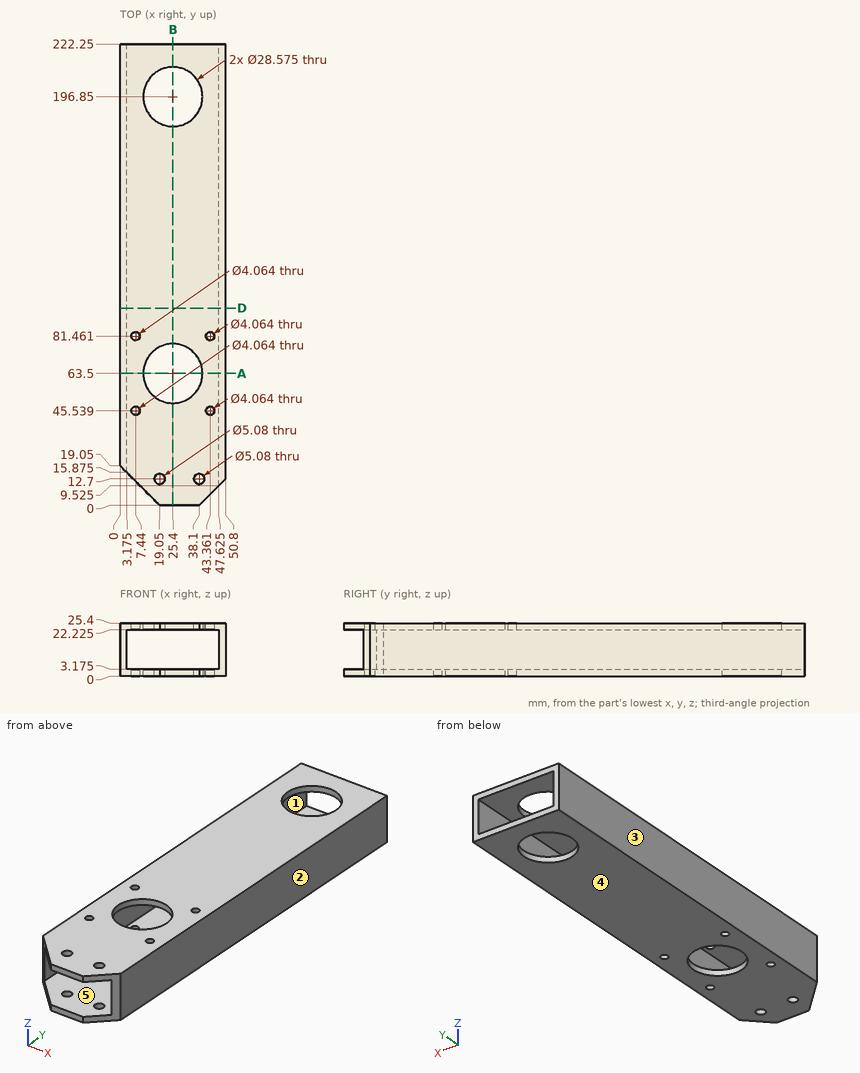
Geometry: see drawing. Coordinates: mm, zero at the bounding-box minimum. A direction names the side the tool comes from. Round coordinates to 2 decimals unless told otherwise and drop trailing zeros. Loops run counter-clockwise (first coordinate to the right, second up) from the corner with the lowest first, then second, coordinate; pieces in that order, holes last. Notation, with made-up numbers: M -22,8.25 L -2,8.25 A21 cw -2,23.25 Z; hole C -10.75,4.25 d1. An arc over 180 degrees is marked long. Use a Markdown table: item, result. Add a question column.
1. Cut plane D-D, the plane y = 95. Output: boundary loops of the cut face in (x, z) (1 decimal).
2. Set-up query: the marked faces 1 and 2. Return all of +Z, -Z, +X, -X, +Y, -Y with unobstructed straight access to the full face (end or side cutting, diameter ignored); none if empty.
3. Contact query for a flat-ended pin moving along its axis: pin 1 (3 mm diameter, centred on x = 44, z = 6.5, fed in from +Y). Output: stop coordinate, or through.
4. Cut plane A-A, the plane y = 63.5. Output: boundary loops of the cut face in (x, z) (1 decimal), and give its area (3 significant figures).
5. Pull-direction query (X, two-part tool) for the marked faces 3, 4 and 5; classes: +X half, -X half, draft (parallel to the pull), parting line (faces both ways), or undercut.
6. Cut plane B-B, the plane x = 25.4. State how many separate pieces and enclosed holes the cut face has, and give its area (3 significant figures).
7. Ray query, line 1 along Z through (x, y) = (6, 137.5) (1 decimal); line 2 along Y through (x, z) = (25.4, 22.9); line 3 along X through (y, z) = (158, 12.5) (1 decimal). Return the intervals inside material, ascending. Write a range as [from, to].
Solution:
| question | item | result |
|---|---|---|
| 1 | outline | M 0,0 L 50.8,0 L 50.8,25.4 L 0,25.4 Z; hole M 3.2,3.2 L 47.6,3.2 L 47.6,22.2 L 3.2,22.2 Z |
| 2 | face 1 | +Y, -Y |
| 2 | face 2 | +Z, -Z, +X, +Y, -Y |
| 3 | pin 1 | passes through |
| 4 | outline | M 0,0 L 11.1,0 L 11.1,3.2 L 3.2,3.2 L 3.2,22.2 L 11.1,22.2 L 11.1,25.4 L 0,25.4 Z; M 39.7,0 L 50.8,0 L 50.8,25.4 L 39.7,25.4 L 39.7,22.2 L 47.6,22.2 L 47.6,3.2 L 39.7,3.2 Z |
| 4 | area | 262 mm2 |
| 5 | face 3 | -X half |
| 5 | face 4 | draft |
| 5 | face 5 | undercut |
| 6 | separate pieces | 6 |
| 6 | enclosed holes | 0 |
| 6 | area | 1,050 mm2 |
| 7 | line 1 | z = [0, 3.2], [22.2, 25.4] |
| 7 | line 2 | y = [0, 49.21], [77.79, 182.56], [211.14, 222.25] |
| 7 | line 3 | x = [0, 3.2], [47.6, 50.8] |
